Input: part model. Units: mm. Frame: model coordinates. Face numbers are marked on the shaded views. A direction names the side the tool comes from. Round coordinates to 2 decimals unless told otherwise and drop trailing zeros. Loops run counter-clockwise (first coordinate to the right, second up) from the corner with the lowest first, then second, coordinate; pieces in that order, holes last.
1) Access query for the marked faces 1 and 2. Directions: +Z, -Z, +X, -X, +Y, -Y. A direction counts if a zero-diameter tool reaches every point of the face in a straight line with its end or side. Return the directions, or none.
2) Section C-C, the plane y = 27.5. Return loops of the section in (x, z).
3) Section D-D, the plane x = 69. Return loops of the section in (y, z), and give its area (3 significant figures).
4) Ray query, line 1 along Y through (x, z) = (46.5, -3.5); line 2 along X through (y, z) = (85, -3.5); line 3 along X through (y, z) = (19, 1). Return the intervals inside material, ascending.
5) Section B-B, the plane y = 63.5. Return loops of the section in (x, z).
6) Section A-A, the plane x = -3. Return loops of the section in (y, z).
7) First-contact query: pin 1 (3 mm diameter, centred on x = 75, y = 44.5, fed in from +Z); pin 2 (2.5 mm diameter, centred on x = 69.5, y = 93, fed in from +Z); pin 3 (4 mm diameter, centred on x = 36.5, z = 11, fed in from -Y). Flat tips, straight axial feed; report the tip coordinate or a pass-through.
8) Draft query along Y for the marked faces 3, 4, 5 and 6. Return one class per face: pulls with the +Y half, pulls with the -Y half, needs draft (parallel to the pull), parting line crosses it, or undercut.
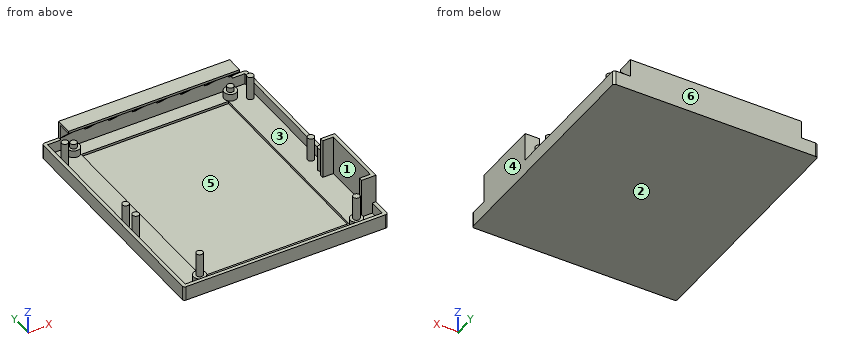
from build123d import *

# Parameters (mm, degrees)
SKETCH002_W            = 100
SKETCH002_H            = 1.5
PAD001_DEPTH           = 79
PAD001_DEPTH_BACK      = 7
SKETCH004_R            = 2.6
PAD003_DEPTH           = 3
SKETCH007_W            = 29
SKETCH007_H            = 1.5
PAD006_DEPTH           = 16.6
SKETCH008_W            = 29
SKETCH008_H            = 16.6
PAD007_DEPTH           = 4.5
SKETCH009_W            = 26
SKETCH009_H            = 16.6
POCKET001_DEPTH        = 10
SKETCH010_W            = 85
SKETCH010_H            = 62
POCKET002_DEPTH        = 1
PAD009_DEPTH           = 4.6
SKETCH019_W            = 1.5
SKETCH019_H            = 72
PAD015_DEPTH           = 6.5
PAD016_DEPTH           = 1.5
LINEARPATTERN_COUNT    = 8
LINEARPATTERN_PITCH    = 10.071429
SKETCH021_W            = 7
SKETCH021_H            = 72
PAD017_DEPTH           = 1
SKETCH022_R            = 1.4
SKETCH022_R_2          = 1.37
PAD023_DEPTH           = 2
SKETCH029_R            = 1.37
PAD024_DEPTH           = 10
SKETCH031_R            = 1.37
PAD026_DEPTH           = 10
FILLET001_R            = 1
LINEARPATTERN001_COUNT = 2
LINEARPATTERN001_PITCH = 42.8
SKETCH036_R            = 1.37
PAD029_DEPTH           = 10


with BuildPart() as part:
    # Sketch002 → Pad001 (new body, two sides)
    with BuildSketch(Plane.YZ) as pad001_sk:
        with Locations((47.5, -3.75)):
            Rectangle(SKETCH002_W, SKETCH002_H)
    extrude(amount=PAD001_DEPTH)
    extrude(pad001_sk.sketch, amount=-PAD001_DEPTH_BACK)

    # Sketch004 (on Face1 of Pad001) → Pad003 (join)
    with BuildSketch(Plane(origin=(0, 0, -3), x_dir=(0, -1, 0), z_dir=(0, 0, 1))):
        with Locations((-3, 3)):
            Circle(SKETCH004_R)
        with Locations((-3, 69)):
            Circle(SKETCH004_R)
        with Locations((-92, 3)):
            Circle(SKETCH004_R)
        with Locations((-92, 69)):
            Circle(SKETCH004_R)
    extrude(amount=PAD003_DEPTH)

    # Sketch007 (on Face1 of Pad003) → Pad006 (join)
    with BuildSketch(Plane(origin=(0, 0, -3), x_dir=(0, -1, 0), z_dir=(0, 0, 1))):
        with Locations((-20.5, 78.25)):
            Rectangle(SKETCH007_W, SKETCH007_H)
    extrude(amount=PAD006_DEPTH)

    # Sketch008 (on Face6 of Pad006) → Pad007 (join)
    with BuildSketch(Plane(origin=(77.5, 0, 0), x_dir=(0, 1, 0), z_dir=(-1, 0, 0))):
        with Locations((20.5, -5.3)):
            Rectangle(SKETCH008_W, SKETCH008_H)
    extrude(amount=PAD007_DEPTH)

    # Sketch009 (on Face6 of Pad006) → Pocket001 (cut)
    with BuildSketch(Plane(origin=(77.5, 0, 0), x_dir=(0, 1, 0), z_dir=(-1, 0, 0))):
        with Locations((20.5, -5.3)):
            Rectangle(SKETCH009_W, SKETCH009_H)
    extrude(amount=POCKET001_DEPTH, mode=Mode.SUBTRACT)

    # Sketch010 (on Face1 of Pocket001) → Pocket002 (cut)
    with BuildSketch(Plane(origin=(0, 0, -3), x_dir=(0, -1, 0), z_dir=(0, 0, 1))):
        with Locations((-47.5, 36)):
            Rectangle(SKETCH010_W, SKETCH010_H)
    extrude(amount=-POCKET002_DEPTH, mode=Mode.SUBTRACT)

    # Sketch012 (on Face1 of Pocket002) → Pad009 (join)
    with BuildSketch(Plane(origin=(0, 0, -3), x_dir=(0, -1, 0), z_dir=(0, 0, 1))):
        Polygon((-35, 79), (-35, 77.5), (-96, 77.5), (-96, -5.5), (1, -5.5), (1, 77.5), (-6, 77.5), (-6, 79), (2.5, 79), (2.5, -7), (-97.5, -7), (-97.5, 79), align=None)
    extrude(amount=PAD009_DEPTH)

    # Sketch019 (on Face20 of Pad009) → Pad015 (join)
    with BuildSketch(Plane(origin=(0, 0, 1.6), x_dir=(0, -1, 0), z_dir=(0, 0, 1))):
        with Locations((-96.75, 36)):
            Rectangle(SKETCH019_W, SKETCH019_H)
    extrude(amount=PAD015_DEPTH)

    # Sketch020 (on Face41 of Pad015) → Pad016 (join)
    with BuildSketch(Plane.YZ.offset(72)):
        Polygon((96, 8.1), (96, 2.6), (90.5, 8.1), align=None)
    pad016 = extrude(amount=-PAD016_DEPTH)

    # LinearPattern: Pad016 ×8
    with Locations(*[(-i * LINEARPATTERN_PITCH, 0, 0) for i in range(1, LINEARPATTERN_COUNT)]):
        add(pad016)

    # Sketch021 (on Face44 of LinearPattern) → Pad017 (join)
    with BuildSketch(Plane(origin=(0, 0, 8.1), x_dir=(0, -1, 0), z_dir=(0, 0, 1))):
        with Locations((-94, 36)):
            Rectangle(SKETCH021_W, SKETCH021_H)
    extrude(amount=PAD017_DEPTH)

    # Sketch022 (on Face31 of Pad017) → Pad023 (join)
    with BuildSketch(Plane(origin=(0, 0, 0), x_dir=(0, -1, 0), z_dir=(0, 0, 1))):
        with Locations((-92, 69)):
            Circle(SKETCH022_R)
        with Locations((-92, 3)):
            Circle(SKETCH022_R_2)
    extrude(amount=PAD023_DEPTH)

    # Sketch029 (on Face32 of Pad023) → Pad024 (join)
    with BuildSketch(Plane(origin=(0, 0, 0), x_dir=(0, -1, 0), z_dir=(0, 0, 1))):
        with Locations((-3, 69)):
            Circle(SKETCH029_R)
        with Locations((-3, 3)):
            Circle(SKETCH029_R)
    extrude(amount=PAD024_DEPTH)

    # Sketch031 (on Face1 of Pad024) → Pad026 (join)
    with BuildSketch(Plane(origin=(0, 0, -3), x_dir=(0, -1, 0), z_dir=(0, 0, 1))):
        with Locations((-88, -3)):
            Circle(SKETCH031_R)
        with Locations((-88, 75)):
            Circle(SKETCH031_R)
    pad026 = extrude(amount=PAD026_DEPTH)

    # Fillet001
    fillet001_edges = [part.edges().sort_by_distance(p)[0] for p in [
        (79, 97.5, -0.7),
        (-7, 97.5, -0.7),
        (-7, -2.5, -0.7),
        (79, -2.5, -0.7),
    ]]
    fillet(fillet001_edges, radius=FILLET001_R)

    # LinearPattern001: Pad026 ×2
    with Locations(*[(0, -i * LINEARPATTERN001_PITCH, 0) for i in range(1, LINEARPATTERN001_COUNT)]):
        add(pad026)

    # Sketch036 (on Face21 of LinearPattern001) → Pad029 (join)
    with BuildSketch(Plane(origin=(0, 0, -3), x_dir=(0, -1, 0), z_dir=(0, 0, 1))):
        with Locations((-38, 75)):
            Circle(SKETCH036_R)
        with Locations((-38, -3)):
            Circle(SKETCH036_R)
    extrude(amount=PAD029_DEPTH)


solid = part.part
Final values:
1. face 1: +Z
1. face 2: -Z, +X, -X, +Y, -Y
2. outline: (-7, -4.5) - (79, -4.5) - (79, 13.6) - (77.5, 13.6) - (77.5, -3) - (67, -3) - (67, -4) - (5, -4) - (5, -3) - (-5.5, -3) - (-5.5, 1.6) - (-7, 1.6) - close
3. outline: (-2.5, -4.5) - (97.5, -4.5) - (97.5, 9.1) - (90.5, 9.1) - (90.5, 8.1) - (96, 8.1) - (96, -3) - (94.6, -3) - (94.6, 0) - (93.4, 0) - (93.4, 2) - (90.6, 2) - (90.6, 0) - (89.4, 0) - (89.4, -3) - (5.6, -3) - (5.6, 0) - (4.37, 0) - (4.37, 10) - (1.63, 10) - (1.63, 0) - (0.4, 0) - (0.4, -3) - (-1, -3) - (-1, 1.6) - (-2.5, 1.6) - close
3. area: 245 mm2
4. line 1: y = -2.5 to 5, 90 to 97.5
4. line 2: x = -7 to 5, 67 to 79
4. line 3: x = -7 to -5.5, 77.5 to 79
5. outline: (-7, -4.5) - (79, -4.5) - (79, 1.6) - (77.5, 1.6) - (77.5, -3) - (67, -3) - (67, -4) - (5, -4) - (5, -3) - (-5.5, -3) - (-5.5, 1.6) - (-7, 1.6) - close
6. outline: (-2.5, -4.5) - (97.5, -4.5) - (97.5, 1.6) - (96, 1.6) - (96, -3) - (89.37, -3) - (89.37, 7) - (86.63, 7) - (86.63, -3) - (46.57, -3) - (46.57, 7) - (43.83, 7) - (43.83, -3) - (39.37, -3) - (39.37, 7) - (36.63, 7) - (36.63, -3) - (-1, -3) - (-1, 1.6) - (-2.5, 1.6) - close
7. pin 1: stops at z = 7
7. pin 2: stops at z = 9.1
7. pin 3: stops at y = 90.5
8. face 3: undercut
8. face 4: needs draft
8. face 5: undercut
8. face 6: pulls with the +Y half
